Autodesk Inventor part; units mm, degrees
ref_plane "Work Plane1" through (0, 4, 0) normal (0, 1, 0) x (-1, 0, 0)
ref_plane "Work Plane2" through (-17.25, 0, -8.5) normal (1, 0, 0) x (0, 0, -1)
ref_plane "YZ Plane" through (0, 0, 0) normal (1, 0, 0) x (0, 1, 0)
sketch "Sketch1" plane through (0, 0, 0) normal (0, 1, 0) x (-1, 0, 0)
  line L0 (0, 0) -> (23, 0)
  line L1 (23, 0) -> (23, -20.5)
  line L2 (7.5, -28) -> (0, -28)
  line L3 (0, -28) -> (0, 0)
  line L4 (7.5, -28) -> (7.5, -20.5)
  line L5 (7.5, -20.5) -> (23, -20.5)
  line L6 (19, -20.5) -> (19, -16.5)
  line L7 (19, -16.5) -> (20.25, -16.5)
  line L8 (20.25, -16.5) -> (20.25, -13.5)
  line L9 (20.25, -13.5) -> (19, -13.5)
  line L10 (19, -13.5) -> (19, -8.5)
  line L11 (19, -8.5) -> (15.5, -8.5)
  line L12 (15.5, -8.5) -> (15.5, -13.5)
  line L13 (15.5, -13.5) -> (14.25, -13.5)
  line L14 (14.25, -13.5) -> (14.25, -16.5)
  line L15 (14.25, -16.5) -> (15.5, -16.5)
  line L16 (15.5, -20.5) -> (15.5, -16.5)
  line L17 (17.25, -8.5) -> (17.25, -20.5) construction
  dimension "d0" = 28
  dimension "d1" = 23
  dimension "d2" = 7.5
  dimension "d3" = 20.5
  dimension "d4" = 3.5
  dimension "d5" = 6
  dimension "d6" = 4
  dimension "d7" = 3
  dimension "d8" = 5
  dimension "d9" = 4
extrude "Extrusion1" add sketch "Sketch1" along normal blind 8 contours L0 L1 L5 L6 L7 L8 L9 L10 L11 L12 L13 L14 L15 L16 L4 L2 L3
sketch "Sketch2" plane through (0, 8, 0) normal (0, 1, 0) x (1, 0, 0)
  line L0 (0, 0) -> (0, 28) construction
  line L1 (0, 28) -> (-7.5, 28) construction
  line L2 (-7.5, 28) -> (-7.5, 20.5) construction
  line L3 (-7.5, 20.5) -> (-15.5, 20.5) construction
  line L4 (-15.5, 20.5) -> (-15.5, 16.5) construction
  line L5 (-15.5, 16.5) -> (-14.25, 16.5) construction
  line L6 (-14.25, 16.5) -> (-14.25, 13.5) construction
  line L7 (-14.25, 13.5) -> (-15.5, 13.5) construction
  line L8 (-15.5, 13.5) -> (-15.5, 8.5) construction
  line L9 (-15.5, 8.5) -> (-19, 8.5) construction
  line L10 (-19, 8.5) -> (-19, 13.5) construction
  line L11 (-19, 13.5) -> (-20.25, 13.5) construction
  line L12 (-20.25, 13.5) -> (-20.25, 16.5) construction
  line L13 (-20.25, 16.5) -> (-19, 16.5) construction
  line L14 (-19, 16.5) -> (-19, 20.5) construction
  line L15 (-19, 20.5) -> (-23, 20.5) construction
  line L16 (-23, 20.5) -> (-23, 0) construction
  line L17 (-23, 0) -> (0, 0) construction
  point P0 (-12, 7.5)
  point P1 (-3, 7.5)
  dimension "d12" = 7.5
  dimension "d13" = 3
  dimension "d14" = 9
hole "Hole1" at (-12, 8, -7.5) at (-3, 8, -7.5) direction (0, -1, 0) diameter 2 end through all
fillet "Fillet1" radius 2 2 edges at (-23, 4, 0) (0, 4, 0)
ref_plane "Work Plane1" through (0, 4, 0) normal (0, 1, 0) x (-1, 0, 0)
ref_plane "Work Plane2" through (-17.25, 0, -8.5) normal (1, 0, 0) x (0, 0, -1)
equation "\"d23\" = 0.5 * THICKNESS"
properties part number "A8-0018"
Could you check a few things on this model? Use its own coordinates, in mm. A direction names the side the tool comes from. Coordinates: 2 decimals unless noted, no trailing zeros. Write each loop counter-clockwise with the first axis right and the second up, starting at its lowest first coordinate (ties: lowest second). Pieces come first, ordered by that corner, then holes. Notation, with made-up numbers: M -16,55.5 L 15,55.5 A19 ccw 15,91.5 Z; hole C -32,-31.75 d6. An arc over 180 degrees is marked long. Answer as CSV lines item,"result". Start each with the question number.
1) I want a section at D-D, the plane x = -3. Please give me the cut outline in (y, z).
2) I want a section at A-A, the plane z = -7.5. Please give me the cut outline in (x, y).
3) For P1, Ø1.4, axis at x = -19.5, y = 5, coming from the -Z side, with a flat end and sliding along its axis, tell me the tip position at first contact or that it passes through.
4) I want a section at B-B, the plane x = -12. Please give me the cut outline in (y, z), and give its area (3 significant figures).
5) We'd pull the mould along Z, two halves only. Please class faces 1 (the flat face through (-20, 4, -16.5)), 2 (the flat face through (-11, 4, -20.5)), 3 (the flat face through (-23, 4, -11)): +Z half, -Z half, draft (parallel to the pull), parting line (faces both ways), or undercut.
6) I want a section at C-C, the plane y = 0.5. Please give me the cut outline in (x, z), and give its area (3 significant figures).
7) Please list where these lines run through material, in increasing order: line 1 (X direction, y = 3, z = -7.5); line 2 (Z direction, x = -3, y = 2.5); line 3 (X direction, y = 4.25, z = -18.25). Write a range as from..to.
8) For faces 4 (the flat face through (-15.5, 4, -11)), 5 (the flat face through (-20.25, 4, -15)), 6 (the cylindrical face through (-22.43, 4.06, -0.6)), 7 (the flat face through (-21, 4, -20.5)), which set-ups out of +Z, -Z, +X, -X, +Y, -Y let a thin tool reach every point of the face, with its end or its side?
Data:
1,outline,"M 0,-28 L 8,-28 L 8,-8.5 L 0,-8.5 Z; M 0,-6.5 L 8,-6.5 L 8,0 L 0,0 Z"
2,outline,"M -23,0 L -13,0 L -13,8 L -23,8 Z; M -11,0 L -4,0 L -4,8 L -11,8 Z; M -2,0 L 0,0 L 0,8 L -2,8 Z"
3,P1,"stops at z = -20.5"
4,outline,"M 0,-20.5 L 8,-20.5 L 8,-8.5 L 0,-8.5 Z; M 0,-6.5 L 8,-6.5 L 8,0 L 0,0 Z"
4,area,"148 mm^2"
5,face 1,"undercut"
5,face 2,"-Z half"
5,face 3,"draft"
6,outline,"M -23,-20.5 L -19,-20.5 L -19,-16.5 L -20.25,-16.5 L -20.25,-13.5 L -19,-13.5 L -19,-8.5 L -15.5,-8.5 L -15.5,-13.5 L -14.25,-13.5 L -14.25,-16.5 L -15.5,-16.5 L -15.5,-20.5 L -7.5,-20.5 L -7.5,-28 L 0,-28 L 0,-2 A2 ccw -2,0 L -21,0 A2 ccw -23,-2 Z; hole C -12,-7.5 d2; hole C -3,-7.5 d2"
6,area,"470 mm^2"
7,line 1,"x = -23..-13, -11..-4, -2..0"
7,line 2,"z = -28..-8.5, -6.5..0"
7,line 3,"x = -23..-19, -15.5..0"
8,face 4,"-Z, +Y, -Y"
8,face 5,"+Y, -Y"
8,face 6,"+Z, -X, +Y, -Y"
8,face 7,"-Z, -X, +Y, -Y"
